The model under review builds one solid part; all positions refer to its coordinate system, in mm. Face numbers are marked on the shaded views. Round coordinates to 2 decimals unless told otherwise and drop trailing zeros. Order: outer loops, then holes, each group sorted by start corner. A loop starts at its lowest first (then second) coordinate and runs counter-clockwise, first axis right, second up.
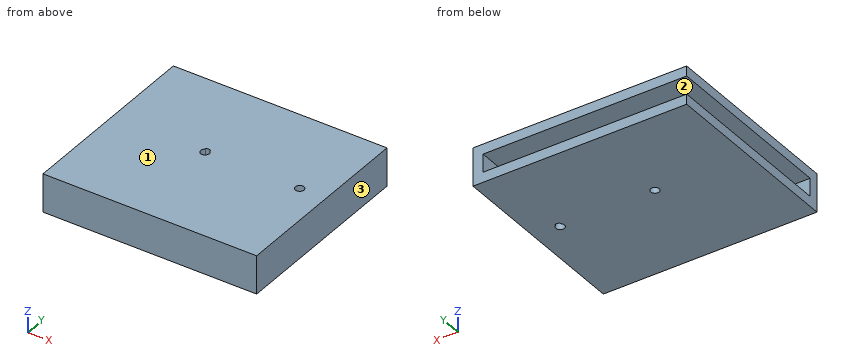
```python
from build123d import *

# Parameters (mm, degrees)
SKETCH1_W           = 101
SKETCH1_H           = 90
BOSS_EXTRUDE1_DEPTH = 5
SKETCH2_W           = 14
SKETCH2_H           = 90
BOSS_EXTRUDE2_DEPTH = 5
SKETCH3_W           = 106
SKETCH3_H           = 90
BOSS_EXTRUDE3_DEPTH = 5
SKETCH4_W           = 106
SKETCH4_H           = 19
BOSS_EXTRUDE4_DEPTH = 5
SKETCH5_R           = 2.15
CUT_EXTRUDE1_DEPTH  = 20
CUT_EXTRUDE2_DEPTH  = 10
CUT_EXTRUDE3_DEPTH  = 10


with BuildPart() as part:
    # Sketch1 → Boss-Extrude1 (new body)
    with BuildSketch(Plane.XY):
        with Locations((30.353658537, 10.426829268)):
            Rectangle(SKETCH1_W, SKETCH1_H)
    extrude(amount=BOSS_EXTRUDE1_DEPTH)

    # Sketch2 → Boss-Extrude2 (add)
    with BuildSketch(Plane(origin=(80.853658537, 0, 0), x_dir=(0, 0, -1), z_dir=(1, 0, 0))):
        with Locations((2, 10.426829268)):
            Rectangle(SKETCH2_W, SKETCH2_H)
    extrude(amount=BOSS_EXTRUDE2_DEPTH)

    # Sketch3 → Boss-Extrude3 (add)
    with BuildSketch(Plane(origin=(0, 0, -9), x_dir=(-1, 0, 0), z_dir=(0, 0, -1))):
        with Locations((-32.853658537, 10.426829268)):
            Rectangle(SKETCH3_W, SKETCH3_H)
    extrude(amount=BOSS_EXTRUDE3_DEPTH)

    # Sketch4 → Boss-Extrude4 (add)
    with BuildSketch(Plane.XZ.offset(34.573170732)):
        with Locations((32.853658537, -4.5)):
            Rectangle(SKETCH4_W, SKETCH4_H)
    extrude(amount=BOSS_EXTRUDE4_DEPTH)

    # Sketch5 → Cut-Extrude1 (cut, through all)
    with BuildSketch(Plane(origin=(0, 0, -14), x_dir=(-1, 0, 0), z_dir=(0, 0, -1))):
        with Locations((-72.853658537, 10.926829268)):
            Circle(SKETCH5_R)
        with Locations((-25.853658537, 10.926829268)):
            Circle(SKETCH5_R)
    extrude(amount=-CUT_EXTRUDE1_DEPTH, mode=Mode.SUBTRACT)

    # Sketch6 → Cut-Extrude2 (cut)
    with BuildSketch(Plane(origin=(0, 0, -14), x_dir=(-1, 0, 0), z_dir=(0, 0, -1))):
        with BuildLine():
            Line((-72.853658537, 10.926829268), (-71.524860303, 13.138320904))
            ThreePointArc((-71.524860303, 13.138320904), (-72.853658537, 13.506829268), (-74.18245677, 13.138320904))
            Line((-74.18245677, 13.138320904), (-72.853658537, 10.926829268))
        make_face()
    extrude(amount=-CUT_EXTRUDE2_DEPTH, mode=Mode.SUBTRACT)

    # Sketch7 → Cut-Extrude3 (cut)
    with BuildSketch(Plane.XY.offset(5)):
        with BuildLine():
            Line((25.853658537, 10.926829268), (27.18245677, 13.138320904))
            ThreePointArc((27.18245677, 13.138320904), (25.853658537, 13.506829268), (24.524860303, 13.138320904))
            Line((24.524860303, 13.138320904), (25.853658537, 10.926829268))
        make_face()
    extrude(amount=-CUT_EXTRUDE3_DEPTH, mode=Mode.SUBTRACT)


solid = part.part
```
(1) Consider section C-C (y = 40). Write out the cut boundary in (x, z).
Data:
outline: (-20.15, -14) - (85.85, -14) - (85.85, 5) - (-20.15, 5) - (-20.15, 0) - (80.85, 0) - (80.85, -9) - (-20.15, -9) - close
(2) Consider section B-B (z = -7). Write out the cut boundary in (x, y).
Data:
outline: (-20.15, -39.57) - (85.85, -39.57) - (85.85, 55.43) - (80.85, 55.43) - (80.85, -34.57) - (-20.15, -34.57) - close
(3) Consider section A-A (x = 68). Write out the cut boundary in (y, z).
Data:
outline: (-39.57, -14) - (55.43, -14) - (55.43, -9) - (-34.57, -9) - (-34.57, 0) - (55.43, 0) - (55.43, 5) - (-39.57, 5) - close
(4) Insertion check: pin 1 (4 mm diameter, centred on x = 72.85, y = 10.93, fed in from +Z); pin 2 (2.5 mm diameter, centred on x = 26.5, z = -6, fed in from +Y); pin 3 (5.5 mm diameter, centred on x = 25.85, y = 10.93, fed in from +Z); pin 4 (1.5 mm diameter, centred on y = -25.5, z = -2.5, fed in from -X). Each pin has a flat end and moves straight along its axis. Give the tip position at first contact, or say it passes through.
Data:
pin 1: passes through
pin 2: stops at y = -34.57
pin 3: stops at z = 5
pin 4: stops at x = 80.85
(5) To check wall thickness, follow probe 1 along Z at (x, y) = (73.5, -18); probe 2 along X at (y, z) = (-1, -3.5); probe 3 along Y at (x, z) = (-3.5, -5). State the ranges of each line that lie inside material, in increasing order.
Data:
probe 1: z = -14 to -9, 0 to 5
probe 2: x = 80.85 to 85.85
probe 3: y = -39.57 to -34.57
(6) Draft analysis for pull direction Z (two halves, no side actions). For the marked faces 1, 2 and 3, state which applies: pulls with the +Z half, pulls with the -Z half, needs draft (parallel to the pull), parting line crosses it, or undercut.
Data:
face 1: pulls with the +Z half
face 2: undercut
face 3: needs draft
